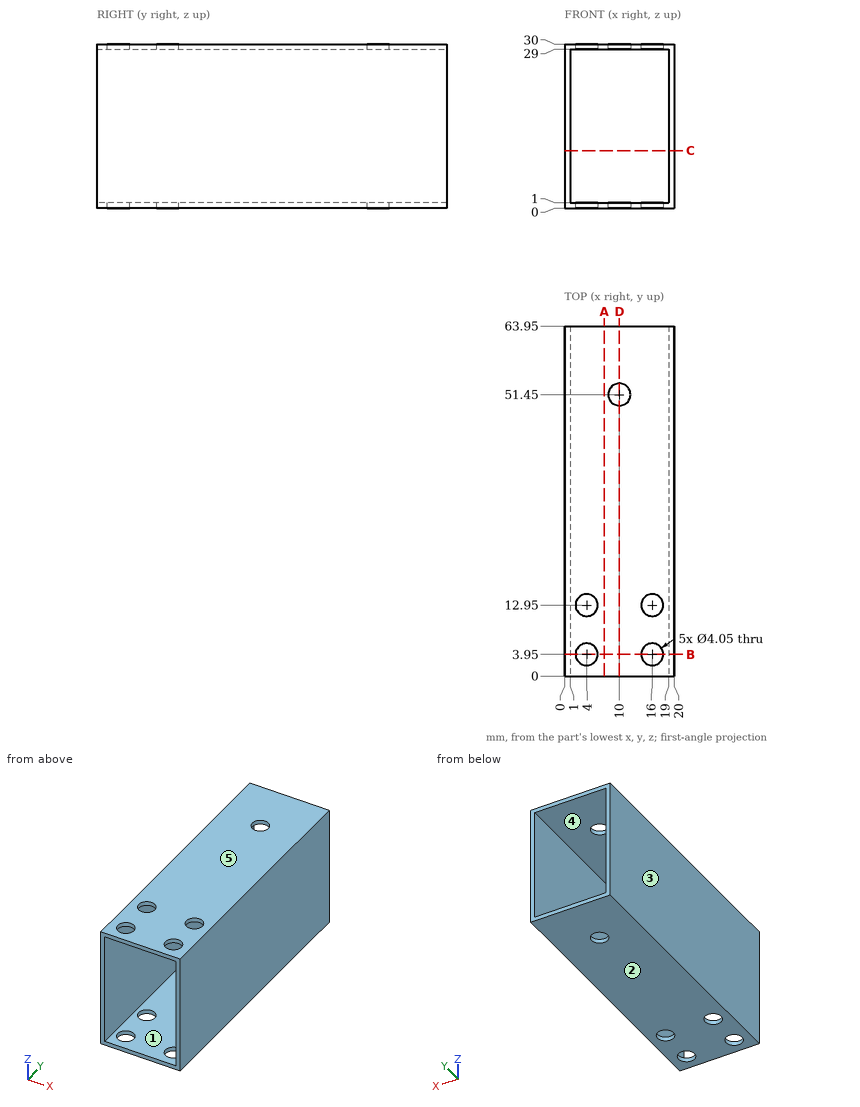
Design review of the part shown in the three views and the two pictorial views. Dimensions are in mm from the part's minimum x, y and z. A direction names the side the tool comes from. Coordinates: 2 decimals unless noted, no trailing zeros. Order: outer loops, then holes, each group sorted by start corner. A loop starts at its lowest first (then second) coordinate and runs counter-clockwise, first axis right, second up. Notation, with made-up numbers: (49.5, -34) - (99.5, -34) arc R16 cw to (99.5, -21) - close; hole circle Ø3 at (-24.5, -19.5). An arc over 180 degrees is marked (long way). Answer as CSV lines item,"result". Start each with the question number.
1) To check wall thickness, follow line 1 along Y through (x, z) = (4, 29.7) (3 decimals); line 2 along X through (y, z) = (5.5, 25.75); line 3 along Z through (x, y) = (6.5, 26). State the ranges of each line that lie inside material, in increasing order. Write a range as [from, to].
2) Add section C-C (z = 10.5). State the section outline as (x, y) points.
3) Add section D-D (x = 10). State the section outline as (y, z) points (3 decimals).
4) Draft analysis for pull direction X (two halves, no side actions). For the marked faces 1, 2 and 3, state which applies: +X half, -X half, draft (parallel to the pull), parting line (faces both ways), or undercut.
5) Add section A-A (x = 7.25). State the section outline as (y, z) points, then the cut area to 3 significant figures.
6) Add section B-B (y = 3.95). State the section outline as (x, z) points (3 decimals).
7) Machinability: for the marked faces 4 and 5, which of the approach directions +Z, -Z, +X, -X, +Y, -Y give a long, thin tool a straight path to every point of the face, cutting with its end or side? Answer none if there is none.
Result:
1,line 1,"[0, 1.925], [5.975, 10.925], [14.975, 63.95]"
1,line 2,"[0, 1], [19, 20]"
1,line 3,"[0, 1], [29, 30]"
2,outline,"(0, 0) - (1, 0) - (1, 63.95) - (0, 63.95) - close; (19, 0) - (20, 0) - (20, 63.95) - (19, 63.95) - close"
3,outline,"(0, 0) - (49.425, 0) - (49.425, 1) - (0, 1) - close; (0, 29) - (49.425, 29) - (49.425, 30) - (0, 30) - close; (53.475, 0) - (63.95, 0) - (63.95, 1) - (53.475, 1) - close; (53.475, 29) - (63.95, 29) - (63.95, 30) - (53.475, 30) - close"
4,face 1,"undercut"
4,face 2,"draft"
4,face 3,"-X half"
5,outline,"(0, 0) - (63.95, 0) - (63.95, 1) - (0, 1) - close; (0, 29) - (63.95, 29) - (63.95, 30) - (0, 30) - close"
5,area,"128 mm^2"
6,outline,"(0, 0) - (1.975, 0) - (1.975, 1) - (1, 1) - (1, 29) - (1.975, 29) - (1.975, 30) - (0, 30) - close; (6.025, 0) - (13.975, 0) - (13.975, 1) - (6.025, 1) - close; (6.025, 29) - (13.975, 29) - (13.975, 30) - (6.025, 30) - close; (18.025, 0) - (20, 0) - (20, 30) - (18.025, 30) - (18.025, 29) - (19, 29) - (19, 1) - (18.025, 1) - close"
7,face 4,"+Y, -Y"
7,face 5,"+Z, +X, -X, +Y, -Y"
